from build123d import *

# Parameters (mm, degrees)
EXTRUDE1_DEPTH  = 340
LPATTERN1_COUNT = 6
LPATTERN1_PITCH = 60


with BuildPart() as part:
    # Sketch1 → Extrude1 (new body)
    with BuildSketch(Plane(origin=(-20, 0, 0), x_dir=(1, 0, 0), z_dir=(0, 0, 1))):
        with BuildLine():
            Line((8.5, 18.910271646), (8.5, 17.079302786))
            Line((8.5, 17.079302786), (8.908405711, 16.67089517))
            ThreePointArc((8.908405711, 16.67089517), (10.269774971, 15.975032022), (10.964333487, 14.612996689))
            Line((10.964333487, 14.612996689), (12.197979513, 13.379350662))
            Line((12.197979513, 13.379350662), (12.197979513, 9.800170422))
            Line((12.197979513, 9.800170422), (8.5, 6.10021925))
            Line((8.5, 6.10021925), (8.5, 1))
            Line((8.5, 1), (9.5, 0))
            Line((9.5, 0), (17.75, 0))
            Line((17.75, 0), (18.25, 0.5))
            Line((18.25, 0.5), (21.75, 0.5))
            Line((21.75, 0.5), (22.25, 0))
            Line((22.25, 0), (30.5, 0))
            Line((30.5, 0), (31.5, 1))
            Line((31.5, 1), (31.5, 6.10021925))
            Line((31.5, 6.10021925), (27.802020487, 9.800170422))
            Line((27.802020487, 9.800170422), (27.802020487, 13.379350662))
            Line((27.802020487, 13.379350662), (29.035666513, 14.612996689))
            ThreePointArc((29.035666513, 14.612996689), (29.730225029, 15.975032022), (31.091594289, 16.67089517))
            Line((31.091594289, 16.67089517), (31.5, 17.079302786))
            Line((31.5, 17.079302786), (31.5, 18.910271646))
            Line((31.5, 18.910271646), (31.091594289, 19.330832529))
            ThreePointArc((31.091594289, 19.330832529), (29.733913517, 20.021041613), (29.035666513, 21.374606084))
            Line((29.035666513, 21.374606084), (28.410271644, 22))
            Line((28.410271644, 22), (11.589728356, 22))
            Line((11.589728356, 22), (10.964333487, 21.374606084))
            ThreePointArc((10.964333487, 21.374606084), (10.266086483, 20.021041613), (8.908405711, 19.330832529))
            Line((8.908405711, 19.330832529), (8.5, 18.910271646))
        make_face()
    extrude(amount=-EXTRUDE1_DEPTH)

    # Sketch2 → Cut-Revolve1 (revolve, cut)
    with BuildSketch(Plane(origin=(0, 0, 0), x_dir=(0, 0, -1), z_dir=(1, 0, 0)), mode=Mode.PRIVATE) as cut_revolve1_sk:
        Polygon((20, 22), (25.5, 22), (25.5, 13), (23.5, 13), (23.5, 0), (20, 0), align=None)
    cut_revolve1 = revolve(cut_revolve1_sk.sketch.rotate(Axis((0, 0, -20), (0, 1, 0)), 180), axis=Axis((0, 0, -20), (0, 1, 0)), mode=Mode.SUBTRACT)

    # LPattern1: Cut-Revolve1 ×6
    with Locations(*[(0, 0, -i * LPATTERN1_PITCH) for i in range(1, LPATTERN1_COUNT)]):
        add(cut_revolve1, mode=Mode.SUBTRACT)


solid = part.part
Work out the finished part from the listing and answer in its coordinate system (mm). A direction names the side the tool comes from. Round coordinates to 2 decimals unless told otherwise and drop trailing zeros. Write each loop counter-clockwise with the first axis right and the second up, starting at its lowest first coordinate (ties: lowest second). Pieces come first, ordered by that corner, then holes. Notation, with made-up numbers: (6.25, 81.25) -> (63.25, 81.25) arc R25 ccw to (63.25, 108.25) -> close; hole circle Ø4 at (51.5, 46.5). An arc over 180 degrees is marked (long way). Answer as CSV lines item,"result". Start each with the question number.
(1) The mould has two halves that part along X. Classify faces 3 (the cylindrical face through (1.05, 6.41, -136.66)), 4 (the flat face through (0, 11, -340)): +X half, -X half, draft (parallel to the pull), parting line (faces both ways), or undercut.
(2) A tool of negligible diameter and unlimited length cuts with its end or side. For faces 1 (the cylindrical face through (1.652, 17.437, -314.754)), 2 (the flat face through (0, 11, 0)), from which of +Z, -Z, +X, -X, +Y, -Y can it reach the whole face along a straight path? Write none if from no direction.
(3) The part is cut by section A-A, the plane z = -157.5. Give the vertices of the cut face in (x, y).
(4) Each of these flat-tipped pins is pushed along its axis until it touches: pin 1 (2 mm diameter, centred on y = 8.5, z = -204, fed in from +X); pin 2 (3.5 mm diameter, centred on x = 2.5, z = -317.5, fed in from +Y); pin 3 (1.8 mm diameter, centred on x = -1, z = -225, fed in from -Y). Where does it stop, or does it pass through?
(5) Find the intervals of material crossed by probe 1 along X at (y, z) = (16.5, -200); probe 2 along X at (y, z) = (18, -80); probe 3 along Y at (x, z) = (-10, -218.5), in increasing order.
Output values:
1,face 3,"undercut"
1,face 4,"draft"
2,face 1,"+Y"
2,face 2,"+Z, +X, -X, +Y, -Y"
3,outline,"(-11.5, 1) -> (-10.5, 0) -> (-2.25, 0) -> (-1.75, 0.5) -> (1.75, 0.5) -> (2.25, 0) -> (10.5, 0) -> (11.5, 1) -> (11.5, 6.1) -> (7.8, 9.8) -> (7.8, 13.38) -> (9.04, 14.61) arc R2.48 cw to (11.09, 16.67) -> (11.5, 17.08) -> (11.5, 18.91) -> (11.09, 19.33) arc R2.48 cw to (9.04, 21.37) -> (8.41, 22) -> (-8.41, 22) -> (-9.04, 21.37) arc R2.48 cw to (-11.09, 19.33) -> (-11.5, 18.91) -> (-11.5, 17.08) -> (-11.09, 16.67) arc R2.48 cw to (-9.04, 14.61) -> (-7.8, 13.38) -> (-7.8, 9.8) -> (-11.5, 6.1) -> close"
4,pin 1,"stops at x = 10.1"
4,pin 2,"stops at y = 13"
4,pin 3,"stops at y = 0.35"
5,probe 1,"x = -10.5 to -5.5, 5.5 to 10.5"
5,probe 2,"x = -11.5 to -5.5, 5.5 to 11.5"
5,probe 3,"y = 0 to 7.6, 16.21 to 19.79"
